Input: part model. Units: mm. Frame: model coordinates. Face numbers are marked on the shaded views. A direction names the side the tool comes from. Round coordinates to 2 decimals unless told otherwise and drop trailing zeros. Loops run counter-clockwise (first coordinate to the right, second up) from the corner with the lowest first, then second, coordinate; pieces in that order, holes last. Notation, with made-up numbers: M -23.75,-30 L 4.25,-30 A28 cw 4.25,4 Z; hole C -20.5,49.25 d5. An arc over 180 degrees is marked long. Put each result on its own line as item: value. Start each with the question number.
1) Section A-A on z = 1.5. Output: boundary loops of the cut face in (x, y), plus the area to 3 significant figures.
2) Section B-B on z = 15. Output: boundary loops of the cut face in (x, y).
3) Line query: probe 1 along X at (y, z) = (-12, 2); probe 2 along X at (y, z) = (-8.25, 1.75); probe 3 along X at (y, z) = (-11, 20.75). Output: solid intervals per line, ascending.
4) Pin query (flat end, axial travel): pin 1 (0.8 mm diameter, centred on x = 23, y = -4.5, fed in from -Z); pin 2 (0.6 mm diameter, centred on y = -5.5, z = 19, fed in from -X); pin 3 (0.6 mm diameter, centred on y = -5.5, z = 0.5, fed in from +X). Return the tip coordinate at first contact, or that it passes through.
5) Section D-D on z = 20.25. Output: boundary loops of the cut face in (x, y), plus the area to 3 significant figures.
6) Draft query along Z for the marked faces 4, 5, 6 and 7. Return one class per face: +Z half, -Z half, draft (parallel to the pull), parting line (faces both ways), or undercut.
7) Reachability of the marked faces 1, 2 and 3 from +Z, -Z, +X, -X, +Y, -Y: full face, straight path, thin tool, end or side. Return the list, or none.
8) Section C-C on x = 10.25. Output: boundary loops of the cut face in (y, z).
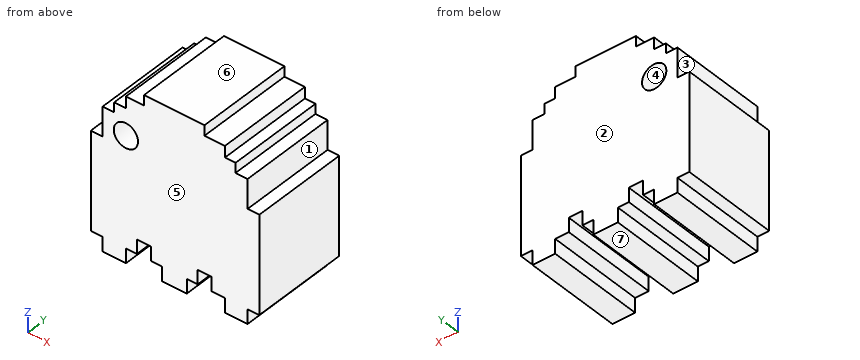
from build123d import *

# Parameters (mm, degrees)
F0_W     = 25.4
F0_H     = 25.4
F1_DEPTH = 12.7
F3_DEPTH = 12.7
F4_R     = 1.5875
F5_DEPTH = 12.7


with BuildPart() as f1:
    # F0 (on Front) → F1 (new body)
    with BuildSketch(Plane.XZ):
        with Locations((12.7, 12.7)):
            Rectangle(F0_W, F0_H)
    extrude(amount=F1_DEPTH)

    # F2 (on face) → F3 (cut)
    with BuildSketch(Plane.XZ.offset(12.7)):
        Polygon((0, 0), (3.20243, 0), (3.20243, 1.880125), (1.660184, 1.880125), (1.660184, 14.615892), (3.20243, 14.615892), (3.20243, 18.416876), (4.726184, 18.416876), (4.726184, 19.700326), (6.249938, 19.700326), (6.249938, 21.18123), (8.620429, 21.18123), (8.620429, 22.514043), (16.518579, 22.514043), (16.518579, 21.18123), (19.184204, 21.18123), (19.184204, 19.700326), (20.566382, 19.700326), (20.566382, 18.416876), (22.146011, 18.416876), (22.146011, 14.615892), (23.676278, 14.615892), (23.676278, 1.880125), (22.146011, 1.880125), (22.146011, 0), (25.4, 0), (25.4, 25.4), (0, 25.4), align=None)
        Polygon((14.198497, 1.880125), (14.198497, 0), (19.184204, 0), (19.184204, 1.880125), (17.407121, 1.880125), (17.407121, 3.706572), (15.630037, 3.706572), (15.630037, 1.880125), align=None)
        Polygon((6.249938, 1.880125), (6.249938, 0), (10.989874, 0), (10.989874, 1.880125), (9.558334, 1.880125), (9.558334, 3.706572), (7.682523, 3.706572), (7.682523, 1.880125), align=None)
    extrude(amount=-F3_DEPTH, mode=Mode.SUBTRACT)

    # F4 (on face) → F5 (cut)
    with BuildSketch(Plane.XZ.offset(12.7)):
        with Locations((6.249938, 16.203392)):
            Circle(F4_R)
    extrude(amount=-F5_DEPTH, mode=Mode.SUBTRACT)


solid = f1.part
Geometry results:
1. outline: M 3.2,-12.7 L 6.25,-12.7 L 6.25,0 L 3.2,0 Z; M 10.99,-12.7 L 14.2,-12.7 L 14.2,0 L 10.99,0 Z; M 19.18,-12.7 L 22.15,-12.7 L 22.15,0 L 19.18,0 Z
1. area: 117 mm²
2. outline: M 3.2,-12.7 L 5.21,-12.7 L 5.21,0 L 3.2,0 Z; M 7.29,-12.7 L 22.15,-12.7 L 22.15,0 L 7.29,0 Z
3. probe 1: x = 1.66 to 7.68, 9.56 to 15.63, 17.41 to 23.68
3. probe 2: x = 3.2 to 6.25, 10.99 to 14.2, 19.18 to 22.15
3. probe 3: x = 6.25 to 19.18
4. pin 1: stops at z = 1.88
4. pin 2: stops at x = 4.73
4. pin 3: stops at x = 22.15
5. outline: M 6.25,-12.7 L 19.18,-12.7 L 19.18,0 L 6.25,0 Z
5. area: 164 mm²
6. face 4: undercut
6. face 5: draft
6. face 6: +Z half
6. face 7: -Z half
7. face 1: +Z, +X, +Y, -Y
7. face 2: +Z, -Z, +X, -X, +Y
7. face 3: +Z, -X, +Y, -Y
8. outline: M -12.7,1.88 L 0,1.88 L 0,22.51 L -12.7,22.51 Z
